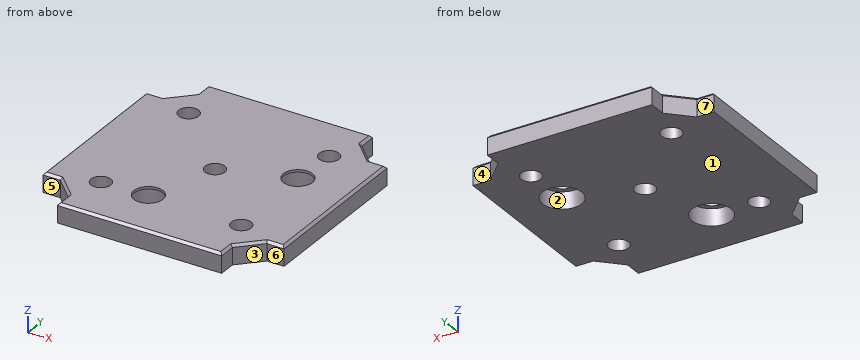
Autodesk Inventor part; units mm, degrees
ref_plane "Work Plane1" through (0, 0, 10) normal (0, 0, 1) x (1, 0, 0)
ref_plane "YZ Plane" through (0, 0, 0) normal (1, 0, 0) x (0, 1, 0)
ref_plane "XZ Plane" through (0, 0, 0) normal (0, 1, 0) x (-1, 0, 0)
ref_plane "Work Plane1" through (0, 0, 10) normal (0, 0, 1) x (1, 0, 0)
sketch "Sketch1" plane through (0, 0, 10) normal (0, 0, 1) x (1, 0, 0)
  line L0 (-4.0299, -0.3538) -> (-2.2322, 1.4439) construction
  arc A0 (-1.4439, 2.2322) -> (-2.2322, 1.4439) centre (-0.9299, 0.9299) ccw construction
  line L1 (-1.4439, 2.2322) -> (0.3538, 4.0299) construction
  line L2 (-37.8299, 42.8299) -> (-37.8299, 37.8299) construction
  line L3 (-37.8299, 37.8299) -> (-42.9208, 37.8299) construction
  line L4 (-37.8299, 42.2137) -> (-37.8299, 45.8299) construction
  line L5 (-37.8299, 45.8299) -> (-4.0299, 45.8299) construction
  line L6 (-4.0299, 45.8299) -> (-4.0299, 42.2137) construction
  line L7 (-4.0299, 4.0299) -> (0.3538, 4.0299)
  circle A1 centre (-20.9299, 20.9299) radius 17.5
  line L8 (-20.9299, 58.9723) -> (17.1124, 20.9299) construction
  line L9 (17.1124, 20.9299) -> (-20.9299, -17.1124) construction
  line L10 (-20.9299, -17.1124) -> (-58.9723, 20.9299) construction
  line L11 (-58.9723, 20.9299) -> (-20.9299, 58.9723) construction
  line L12 (-20.9299, 58.9723) -> (-20.9299, -17.1124) construction
  line L13 (17.1124, 20.9299) -> (-58.9723, 20.9299) construction
  line L14 (-20.9299, 58.9723) -> (32.8701, 58.9723) construction
  line L15 (-43.4299, 43.4299) -> (1.5701, 43.4299) construction
  line L16 (1.5701, 43.4299) -> (1.5701, -1.5701) construction
  line L17 (1.5701, -1.5701) -> (-43.4299, -1.5701) construction
  line L18 (-43.4299, -1.5701) -> (-43.4299, 43.4299) construction
  line L19 (-43.4299, 43.4299) -> (1.5701, -1.5701) construction
  line L20 (1.5701, 43.4299) -> (-43.4299, -1.5701) construction
  line L21 (-43.4299, 5.3876) -> (-43.4299, 36.4723)
  line L22 (-43.4299, 36.4723) -> (-36.4723, 43.4299)
  line L23 (-36.4723, 43.4299) -> (-5.3876, 43.4299)
  line L24 (-5.3876, 43.4299) -> (1.5701, 36.4723)
  line L25 (1.5701, 36.4723) -> (1.5701, 5.3876)
  line L26 (1.5701, 5.3876) -> (-5.3876, -1.5701)
  line L27 (-5.3876, -1.5701) -> (-36.4723, -1.5701)
  line L28 (-36.4723, -1.5701) -> (-43.4299, 5.3876)
  line L29 (-4.0299, 42.2137) -> (-37.8299, 42.2137)
  line L30 (-4.0299, -0.3538) -> (-4.0299, 4.0299)
  circle A2 centre (-20.9299, 20.9299) radius 1.5
  line L31 (-10.9299, 10.9299) -> (-30.9299, 10.9299) construction
  line L32 (-30.9299, 10.9299) -> (-30.9299, 30.9299) construction
  line L33 (-30.9299, 30.9299) -> (-10.9299, 30.9299) construction
  line L34 (-10.9299, 30.9299) -> (-10.9299, 10.9299) construction
  line L35 (-10.9299, 10.9299) -> (-30.9299, 30.9299) construction
  line L36 (-30.9299, 10.9299) -> (-10.9299, 30.9299) construction
  circle A3 centre (-30.9299, 30.9299) radius 1.4
  circle A4 centre (-30.9299, 10.9299) radius 1.4
  circle A5 centre (-10.9299, 10.9299) radius 1.4
  line L37 (-45.8299, 37.8299) -> (-42.0723, 37.8299) construction
  line L38 (-42.1723, 37.7299) -> (-45.8299, 37.7299)
  line L39 (-45.8299, 37.7299) -> (-45.8299, 4.1299)
  line L40 (-45.8299, 4.1299) -> (-42.1723, 4.1299)
  line L41 (-42.1723, 4.1299) -> (-42.1723, 37.7299)
  line L42 (-45.8299, 4.0299) -> (-42.0723, 4.0299) construction
  line L43 (-45.8299, 37.8299) -> (-42.0723, 37.8299)
  line L44 (-37.7299, 45.8299) -> (-4.1299, 45.8299)
  line L45 (-4.1299, 45.8299) -> (-4.1299, 42.1723)
  line L46 (-4.1299, 42.1723) -> (-37.7299, 42.1723)
  line L47 (-37.7299, 42.1723) -> (-37.7299, 45.8299)
  line L48 (0.4701, 37.8299) -> (0.4701, 4.0299) construction
  line L49 (0.4701, 4.0299) -> (3.9701, 4.0299) construction
  line L50 (3.9701, 37.8299) -> (3.9701, 4.0299) construction
  line L51 (0.4701, 37.8299) -> (3.9701, 37.8299) construction
  line L52 (-45.8299, -3.9701) -> (-4.0299, -3.9701) construction
  line L53 (0.3124, 37.7299) -> (3.9701, 37.7299)
  line L54 (3.9701, 37.7299) -> (3.9701, 4.1299)
  line L55 (3.9701, 4.1299) -> (0.3124, 4.1299)
  line L56 (0.3124, 4.1299) -> (0.3124, 37.7299)
  line L57 (-4.1713, -0.3538) -> (-37.7299, -0.3538)
  line L58 (-37.7299, -0.3538) -> (-37.7299, -3.9701)
  line L59 (-37.7299, -3.9701) -> (-4.1713, -3.9701)
  line L60 (-4.1713, -3.9701) -> (-4.1713, -0.3538)
  point P0 (-37.8299, 4.0299)
  dimension "d18" = 53.8
  dimension "d19" = 45
  dimension "d20" = 53.8
  dimension "d21" = 45
  dimension "d22" = 45
  dimension "d30" = 20
  dimension "d31" = 20
  dimension "d32" = 2.8
  dimension "d33" = 2.8
  dimension "d34" = 2.8
  dimension "d35" = 3
  dimension "d36" = 0.1
  dimension "d37" = 0.1
  dimension "d38" = 0.1
  dimension "d39" = 0.1
extrude "Extrusion1" add sketch "Sketch1" along normal blind 10 contours L30 L26 L57 L28 L41 L22 L46 L24 L56 L7 | L7 L26 L30 | L56 L24 L25 L26 | L26 L25 L24 L53 L54 L55 | L60 L59 L58 L57 L28 L27 L26 | L26 L27 L28 L57 | L46 L22 L29 L24 | L24 L29 L45 | L40 L39 L38 L22 L21 L28 | L28 L21 L22 L41 | L29 L22 L23 L24 | L24 L23 L22 L29 L47 L44 L45 | L47 L29 L22 | A1 | A2 | A3 | A4 | A5
sketch "Skizze4" plane through (0, 0, 20) normal (0, 0, 1) x (1, 0, 0)
  line L0 (-37.7299, 42.1723) -> (-42.1723, 37.7299)
  line L1 (-42.1723, 37.7299) -> (-45.8299, 37.7299)
  line L2 (-45.8299, 37.7299) -> (-45.8299, 4.1299) construction
  line L3 (-45.8299, 4.1299) -> (-42.1723, 4.1299)
  line L4 (-42.1723, 4.1299) -> (-37.6885, -0.3538)
  line L5 (-37.6885, -0.3538) -> (-37.7299, -0.3538)
  line L6 (-37.7299, -0.3538) -> (-37.7299, -3.9701)
  line L7 (-37.7299, -3.9701) -> (-4.1713, -3.9701) construction
  line L8 (-4.1713, -3.9701) -> (-4.1713, -0.3538)
  line L9 (-4.1713, -0.3538) -> (0.3124, 4.1299)
  line L10 (0.3124, 4.1299) -> (3.9701, 4.1299)
  line L11 (3.9701, 4.1299) -> (3.9701, 37.7299) construction
  line L12 (3.9701, 37.7299) -> (0.3124, 37.7299)
  line L13 (0.3124, 37.7299) -> (-4.1299, 42.1723)
  line L14 (-4.1299, 42.1723) -> (-4.1299, 45.8299)
  line L15 (-4.1299, 45.8299) -> (-37.7299, 45.8299) construction
  line L16 (-37.7299, 45.8299) -> (-37.7299, 42.1723)
  line L17 (-37.9299, 46.0299) -> (-3.9299, 46.0299) construction
  line L18 (-3.9299, 46.0299) -> (-3.9299, 42.2551)
  line L19 (-3.9299, 42.2551) -> (0.3953, 37.9299)
  line L20 (0.3953, 37.9299) -> (4.1701, 37.9299)
  line L21 (4.1701, 37.9299) -> (4.1701, 3.9299) construction
  line L22 (4.1701, 3.9299) -> (0.3953, 3.9299)
  line L23 (0.3953, 3.9299) -> (-3.9713, -0.4367)
  line L24 (-3.9713, -0.4367) -> (-3.9713, -4.1701)
  line L25 (-3.9713, -4.1701) -> (-37.9299, -4.1701) construction
  line L26 (-37.9299, -4.1701) -> (-37.9299, -0.3953)
  line L27 (-37.9299, -0.3953) -> (-42.2551, 3.9299)
  line L28 (-42.2551, 3.9299) -> (-46.0299, 3.9299)
  line L29 (-46.0299, 3.9299) -> (-46.0299, 37.9299) construction
  line L30 (-46.0299, 37.9299) -> (-42.2551, 37.9299)
  line L31 (-42.2551, 37.9299) -> (-37.9299, 42.2551)
  line L32 (-37.9299, 42.2551) -> (-37.9299, 46.0299)
  line L33 (-45.8299, 37.7299) -> (-45.8299, 37.9299)
  line L34 (-4.1299, 45.8299) -> (-37.7299, 45.8299)
  line L35 (-37.7299, 45.8299) -> (-37.9299, 45.8299)
  line L36 (-4.1299, 45.8299) -> (-3.9299, 45.8299)
  line L37 (3.9701, 37.7299) -> (3.9701, 37.9299)
  line L38 (3.9701, 4.1299) -> (3.9701, 37.7299)
  line L39 (3.9701, 4.1299) -> (3.9701, 3.9299)
  line L40 (-4.1713, -3.9701) -> (-3.9713, -3.9701)
  line L41 (-37.7299, -3.9701) -> (-37.9299, -3.9701)
  line L42 (-45.8299, 4.1299) -> (-45.8299, 3.9299)
  point P0 (0, 0)
  dimension "d40" = 0.2
extrude "IM_offset" add sketch "Skizze4" against normal up to surface (10 mm away)
ref_plane "Work Plane5" through (-37.9299, 20.9299, 10) normal (0, -1, 0) x (1, 0, 0)
ref_plane "Work Plane6" through (-20.9299, 3.9299, 10) normal (1, 0, 0) x (0, 0, -1)
sketch "Sketch24" plane through (0, 0, 10) normal (0, 0, -1) x (-1, 0, 0)
  line L0 (6.4299, 6.4299) -> (35.4299, 6.4299) construction
  line L1 (35.4299, 6.4299) -> (35.4299, 35.4299) construction
  line L2 (35.4299, 35.4299) -> (6.4299, 35.4299) construction
  line L3 (6.4299, 35.4299) -> (6.4299, 6.4299) construction
  line L4 (6.4299, 6.4299) -> (35.4299, 35.4299) construction
  line L5 (35.4299, 6.4299) -> (6.4299, 35.4299) construction
  point P0 (0, 0)
  point P1 (20.9299, 20.9299)
  dimension "d143" = 29
  dimension "d144" = 29
hole "Hole1" at (-20.9299, 20.9299, 10) at (-6.4299, 6.4299, 10) at (-35.4299, 6.4299, 10) at (-35.4299, 35.4299, 10) at (-6.4299, 35.4299, 10) direction (0, 0, 1) diameter 4.1 end through all
sketch "Skizze28" plane through (0, 0, 10) normal (0, 0, -1) x (-1, 0, 0)
  circle A0 centre (25.9299, 6.9299) radius 3
  circle A1 centre (6.9299, 25.9299) radius 3
  line L0 (9.9299, 4.9299) -> (1.9299, 4.9299)
  line L1 (4.9299, 1.9299) -> (1.9299, 4.9299)
  line L2 (36.9299, 1.9299) -> (4.9299, 1.9299)
  line L3 (39.9299, 4.9299) -> (36.9299, 1.9299)
  line L4 (39.9299, 36.9299) -> (39.9299, 4.9299)
  line L5 (36.9299, 39.9299) -> (39.9299, 36.9299)
  line L6 (4.9299, 39.9299) -> (36.9299, 39.9299)
  line L7 (1.9299, 36.9299) -> (4.9299, 39.9299)
  line L8 (1.9299, 8.9299) -> (1.9299, 36.9299)
  line L9 (1.9299, 8.9299) -> (9.9299, 8.9299)
  line L10 (9.9299, 8.9299) -> (9.9299, 4.9299)
  circle A2 centre (34.9299, 6.9299) radius 2
  circle A3 centre (6.9299, 25.9299) radius 4.05
  circle A4 centre (25.9299, 6.9299) radius 4.05
  point P0 (0, 0)
  dimension "d173" = 8.1
  dimension "d174" = 8.1
extrude "Extrusion23" cut sketch "Skizze28" against normal blind 9.5 contours A0 | A1 | A3 | A4
chamfer "Fase2" distance 0.5 angle 45 27 edges at (-2.8799, 25.9299, 10) (-35.4299, 4.3799, 10) (-6.4299, 4.3799, 10) (-20.9299, 18.8799, 10) (-35.4299, 33.3799, 10) (-6.4299, 33.3799, 10) (-21.8799, 6.9299, 10) (-45.8299, 20.9299, 10) (-20.9506, -3.9701, 10) (3.9701, 20.9299, 20) (3.9701, 20.9299, 10) (-20.9299, 45.8299, 10) (-44.0425, 37.9299, 20) (-40.0925, 40.0925, 20) (-37.9299, 44.0425, 20) (-20.9299, 45.8299, 20) (-45.8299, 20.9299, 20) (-44.0425, 3.9299, 20) (-20.9506, -3.9701, 20) (-37.9299, -2.1827, 20) (-40.0925, 1.7673, 20) (-3.9713, -2.2034, 20) (-1.788, 1.7466, 20) (2.1827, 3.9299, 20) (2.1827, 37.9299, 20) (-1.7673, 40.0925, 20) (-3.9299, 44.0425, 20)
sketch "Skizze29" plane through (0, 0, 20) normal (0, 0, 1) x (1, 0, 0)
  circle A0 centre (-35.4299, 6.4299) radius 2.55
  circle A1 centre (-25.9299, 6.9299) radius 4.55
  circle A2 centre (-20.9299, 20.9299) radius 2.55
  circle A3 centre (-6.9299, 25.9299) radius 4.55
  circle A4 centre (-6.4299, 35.4299) radius 2.55
  circle A5 centre (-6.4299, 6.4299) radius 2.55
  circle A6 centre (-35.4299, 35.4299) radius 2.55
  line L0 (3.4701, 4.4299) -> (3.4701, 37.4299)
  line L1 (0.1882, 4.4299) -> (3.4701, 4.4299)
  line L2 (-4.4713, -0.2296) -> (0.1882, 4.4299)
  line L3 (-4.4713, -3.4701) -> (-4.4713, -0.2296)
  line L4 (-37.4299, -3.4701) -> (-4.4713, -3.4701)
  line L5 (-37.4299, -0.1882) -> (-37.4299, -3.4701)
  line L6 (-42.048, 4.4299) -> (-37.4299, -0.1882)
  line L7 (-45.3299, 4.4299) -> (-42.048, 4.4299)
  line L8 (-45.3299, 37.4299) -> (-45.3299, 4.4299)
  line L9 (-42.048, 37.4299) -> (-45.3299, 37.4299)
  line L10 (-37.4299, 42.048) -> (-42.048, 37.4299)
  line L11 (-37.4299, 45.3299) -> (-37.4299, 42.048)
  line L12 (-4.4299, 45.3299) -> (-37.4299, 45.3299)
  line L13 (-4.4299, 42.048) -> (-4.4299, 45.3299)
  line L14 (0.1882, 37.4299) -> (-4.4299, 42.048)
  line L15 (3.4701, 37.4299) -> (0.1882, 37.4299)
  point P0 (0, 0)
hole "Bohrung2" at (-6.9299, 25.9299, 20) at (-25.9299, 6.9299, 20) direction (0, 0, -1) diameter 6 end through all
sketch "Sketch30" plane through (3.9701, 3.9299, 19.5) normal (1, 0, 0) x (0, 0, -1)
  line L0 (9.5, 44.7711) -> (3.5, 44.7711)
  line L1 (3.5, 44.7711) -> (3.5, -17.5234)
  line L2 (3.5, -17.5234) -> (9.5, -17.5234)
  line L3 (9.5, -17.5234) -> (9.5, 44.7711)
  line L4 (9.5, 0.5) -> (9.5, 33.5)
  point P0 (19.5, -3.9299)
  dimension "d187" = 6
extrude "Extrusion24" cut sketch "Sketch30" against normal through all
properties part number "20_Cube_Insert_Kinematic_Mirror_90_pro_magnetic"
Geometry: final body of the model. Coordinates: model frame, mm. Face numbers are marked on the shaded views. A direction names the side the tool comes from. Round coordinates to 2 decimals unless told otherwise and drop trailing zeros. Loops run counter-clockwise (first coordinate to the right, second up) from the corner with the lowest first, then second, coordinate; pieces in that order, holes last. Notation, with made-up numbers: (-28.75, 68.25) -> (4.25, 68.25) arc R33 cw to (4.25, 97.25) -> close; hole circle Ø5 at (34, 44.25). An arc over 180 degrees is marked (long way). Use one line per item in the form item = value. Start each with the question number.
1) Draft query along Y for the marked faces 1, 2 and 3. Return one class per face: released by +Y, released by -Y, zero draft, split by the parting line, or undercut.
2) Section A-A on y = 27.5. Output: boundary loops of the cut face in (x, z).
3) Section B-B on z = 18.05. Output: boundary loops of the cut face in (x, y).
4) Section C-C on y = 2. Output: boundary loops of the cut face in (x, z).
5) Access query for the marked faces 4, 5, 6 and 7. Directions: +Z, -Z, +X, -X, +Y, -Y. A direction counts if a zero-diameter tool reaches every point of the face in a straight line with its end or side. Return the directions, or none.
6) Line query: L1, parallel to X at y = 7, z = 16.2; L2, parallel to Y at x = -10.5, z = 19.2; L3, parallel to Y at x = -9, z = 18.95. Output: solid intervals per line, ascending.
7) First-contact query: P1, Ø1, axis at y = 45, z = 18.5, coming from the +X side; P2, Ø3.5, axis at x = -6.43, y = 6.43, coming from the -Z side; P3, Ø1.8, axis at x = 3, z = 18.5, coming from the -Y side; P4, Ø7, axis at x = -6.93, y = 25.93, coming from the -Z side. Flat tips, straight axial feed; report the tip coordinate or a pass-through.
Response:
q1.face_1 = zero draft
q1.face_2 = undercut
q1.face_3 = released by -Y
q2.outline = (-45.83, 16) -> (-10.66, 16) -> (-10.66, 19.5) -> (-9.49, 19.5) -> (-9.49, 20) -> (-45.33, 20) -> (-45.83, 19.5) -> close; (-4.37, 19.5) -> (-3.2, 19.5) -> (-3.2, 16) -> (3.97, 16) -> (3.97, 19.5) -> (3.47, 20) -> (-4.37, 20) -> close
q3.outline = (-45.83, 3.93) -> (-42.26, 3.93) -> (-37.93, -0.4) -> (-37.93, -3.97) -> (-3.97, -3.97) -> (-3.97, -0.44) -> (0.4, 3.93) -> (3.97, 3.93) -> (3.97, 37.93) -> (0.4, 37.93) -> (-3.93, 42.26) -> (-3.93, 45.83) -> (-37.93, 45.83) -> (-37.93, 42.26) -> (-42.26, 37.93) -> (-45.83, 37.93) -> close; hole circle Ø4.1 at (-35.43, 6.43); hole circle Ø4.1 at (-35.43, 35.43); hole circle Ø8.1 at (-25.93, 6.93); hole circle Ø4.1 at (-20.93, 20.93); hole circle Ø8.1 at (-6.93, 25.93); hole circle Ø4.1 at (-6.43, 6.43); hole circle Ø4.1 at (-6.43, 35.43)
q4.outline = (-40.33, 16) -> (-1.53, 16) -> (-1.53, 19.5) -> (-2.24, 20) -> (-39.62, 20) -> (-40.33, 19.5) -> close
q5.face_4 = +Z, -Z, +X, +Y
q5.face_5 = +Z, -Z, -X, -Y
q5.face_6 = +Z, -Z, +X, -Y
q5.face_7 = +Z, -Z, -X, +Y
q6.L1 = -45.83 to -37.4, -33.46 to -29.98, -21.88 to -8.4, -4.46 to 3.97
q6.L2 = -3.97 to 24.02, 27.84 to 45.83
q6.L3 = -3.97 to 22.45, 29.41 to 45.83
q7.P1 = -3.93
q7.P2 = through
q7.P3 = 3.93
q7.P4 = 19.5
